The listing builds one solid part. Answer for the finished solid, in the listing's coordinates (mm). Give positions to 0.01 mm unless a question says otherwise; leave off trailing zeros. Order: outer loops, then holes, each group sorted by start corner. A loop starts at its lowest first (then second) coordinate and runs counter-clockwise, first axis right, second up. Notation, with made-up numbers: (16.25, 44) - (49.25, 44) arc R19 cw to (49.25, 73) - close; hole circle Ø4 at (46.5, 83). An arc over 180 degrees is marked (long way). Use a Markdown table: item, result. Add a question column.
1) Find section A-A, the plane x = -46.5. Determine the outline of the cut face in (y, z).
2) Find section B-B, the plane z = 1. State how many separate pieces and enclosed holes the cut face has, plus the area to 3 significant figures.
3) Straight lines are drawn through the part: line 1 (Y direction, x = 215, z = 1.1); line 2 (X direction, y = -9, z = 1.7); line 3 (Y direction, x = 0, z = 1.75). For each, find the intervals that lie inside material, in ascending order.
4) Flat-ended cylindrical pins translate along their axes: pin 1 (2.5 mm diameter, centred on x = -83.37, y = -26.74, fed in from -Z); pin 2 (1.5 mm diameter, centred on x = -43, z = 1.5, fed in from +Y). Find the tip coordinate at first contact, or state that the pin passes through.
5) Find section C-C, the plane x = 155. Determine the outline of the cut face in (y, z).
from build123d import *

# Parameters (mm, degrees)
SKETCH1_W           = 458
SKETCH1_H           = 245
BOSS_EXTRUDE1_DEPTH = 3
CUT_EXTRUDE1_DEPTH  = 260.723410574
SKETCH3_R           = 2.5
CUT_EXTRUDE2_DEPTH  = 260.723410574
SKETCH4_R           = 11.5
CUT_EXTRUDE3_DEPTH  = 260.723410574
SKETCH5_W           = 428
SKETCH5_H           = 29
CUT_EXTRUDE4_DEPTH  = 260.723410574
SKETCH8_R           = 1.5
SKETCH8_W           = 69.9
SKETCH8_H           = 41.2
CUT_EXTRUDE5_DEPTH  = 260.723410574
SKETCH9_W           = 458
SKETCH9_H           = 70
CUT_EXTRUDE6_DEPTH  = 10


with BuildPart() as part:
    # Sketch1 → Boss-Extrude1 (new body)
    with BuildSketch(Plane.XY):
        Rectangle(SKETCH1_W, SKETCH1_H)
    extrude(amount=BOSS_EXTRUDE1_DEPTH)

    # Sketch2 → Cut-Extrude1 (cut, through all)
    with BuildSketch(Plane.XY.offset(3)):
        with BuildLine():
            Line((-148, -107.5), (-148, -122.5))
            ThreePointArc((-148, -122.5), (-155, -129.5), (-162, -122.5))
            Line((-162, -122.5), (-162, -107.5))
            ThreePointArc((-162, -107.5), (-155, -100.5), (-148, -107.5))
        make_face()
        with BuildLine():
            Line((162, -107.5), (162, -122.5))
            ThreePointArc((162, -122.5), (155, -129.5), (148, -122.5))
            Line((148, -122.5), (148, -107.5))
            ThreePointArc((148, -107.5), (155, -100.5), (162, -107.5))
        make_face()
    extrude(amount=-CUT_EXTRUDE1_DEPTH, mode=Mode.SUBTRACT)

    # Sketch3 → Cut-Extrude2 (cut, through all)
    with BuildSketch(Plane.XY.offset(3)):
        with Locations((-194, 112.5)):
            Circle(SKETCH3_R)
        with Locations((-194, -107.5)):
            Circle(SKETCH3_R)
        with Locations((194, -107.5)):
            Circle(SKETCH3_R)
        with Locations((194, 112.5)):
            Circle(SKETCH3_R)
        with Locations((-215, 0)):
            Circle(SKETCH3_R)
        with Locations((-215, -90)):
            Circle(SKETCH3_R)
        with Locations((-215, 90)):
            Circle(SKETCH3_R)
        with Locations((215, 0)):
            Circle(SKETCH3_R)
        with Locations((215, -90)):
            Circle(SKETCH3_R)
        with Locations((215, 90)):
            Circle(SKETCH3_R)
        with Locations((0, 112.5)):
            Circle(SKETCH3_R)
        with Locations((0, -107.5)):
            Circle(SKETCH3_R)
    extrude(amount=-CUT_EXTRUDE2_DEPTH, mode=Mode.SUBTRACT)

    # Sketch4 → Cut-Extrude3 (cut, through all)
    with BuildSketch(Plane.XY.offset(3)):
        with Locations((-39, 91)):
            Circle(SKETCH4_R)
        with Locations((39, 91)):
            Circle(SKETCH4_R)
    extrude(amount=-CUT_EXTRUDE3_DEPTH, mode=Mode.SUBTRACT)

    # Sketch5 → Cut-Extrude4 (cut, through all)
    with BuildSketch(Plane.XY.offset(3)):
        with Locations((0, 53)):
            Rectangle(SKETCH5_W, SKETCH5_H)
    extrude(amount=-CUT_EXTRUDE4_DEPTH, mode=Mode.SUBTRACT)

    # Sketch8 → Cut-Extrude5 (cut, through all)
    with BuildSketch(Plane.XY.offset(3)):
        with Locations((5.296172264, 15.703565509)):
            Circle(SKETCH8_R)
        with Locations((5.679687501, -26.054673392)):
            Circle(SKETCH8_R)
        with Locations((-83.3, 14.88)):
            Circle(SKETCH8_R)
        with Locations((-83.367997673, -26.737946691)):
            Circle(SKETCH8_R)
        with Locations((-39, -5.5)):
            Rectangle(SKETCH8_W, SKETCH8_H)
    extrude(amount=-CUT_EXTRUDE5_DEPTH, mode=Mode.SUBTRACT)

    # Sketch9 → Cut-Extrude6 (cut)
    with BuildSketch(Plane.XY.offset(3)):
        with Locations((0, 87.5)):
            Rectangle(SKETCH9_W, SKETCH9_H)
    extrude(amount=-CUT_EXTRUDE6_DEPTH, mode=Mode.SUBTRACT)


solid = part.part
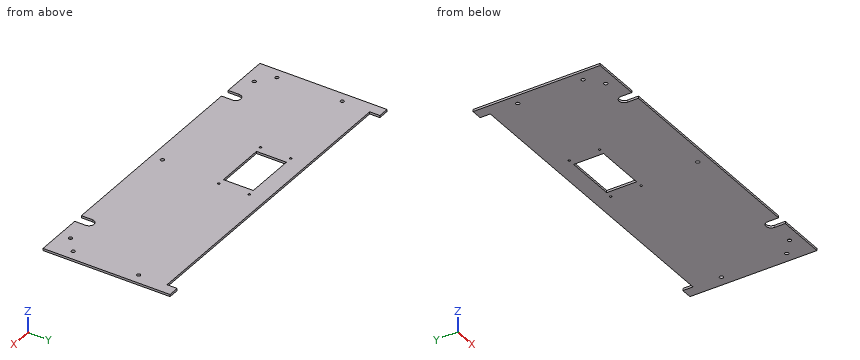
The answers:
| question | item | result |
|---|---|---|
| 1 | outline | (-122.5, 0) - (-26.1, 0) - (-26.1, 3) - (-122.5, 3) - close; (15.1, 0) - (38.5, 0) - (38.5, 3) - (15.1, 3) - close |
| 2 | separate pieces | 1 |
| 2 | enclosed holes | 12 |
| 2 | area | 70,500 mm2 |
| 3 | line 1 | -122.5 to -92.5, -87.5 to -2.5, 2.5 to 52.5 |
| 3 | line 2 | -229 to -73.95, -4.05 to 229 |
| 3 | line 3 | -122.5 to -110, -105 to 38.5 |
| 4 | pin 1 | through |
| 4 | pin 2 | y = 38.5 |
| 5 | outline | (-100.5, 0) - (38.5, 0) - (38.5, 3) - (-100.5, 3) - close |
